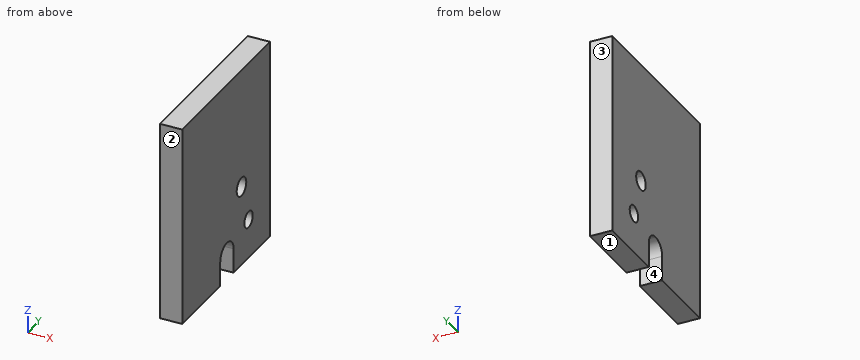
from build123d import *

# Parameters (mm, degrees)
SKETCH_1_W      = 5
SKETCH_1_H      = 5
SKETCH_1_R      = 1.1
EXTRUDE_1_DEPTH = 3
SKETCH_2_W      = 2.809830056
SKETCH_2_H      = 3.158804736
SKETCH_2_H_2    = 9.934341015
EXTRUDE_2_DEPTH = 3


with BuildPart() as part:
    # 草图1 → 凸台-拉伸1 (new body)
    with BuildSketch(Plane(origin=(0, 0, 0), x_dir=(0, 0, -1), z_dir=(1, 0, 0))):
        with Locations((2.5, -2.5)):
            Rectangle(SKETCH_1_W, SKETCH_1_H)
        with Locations((2.5, -2.5)):
            Circle(SKETCH_1_R, mode=Mode.SUBTRACT)
    extrude(amount=EXTRUDE_1_DEPTH)

    # 草图2 → 凸台-拉伸2 (add)
    with BuildSketch(Plane.ZY):
        with Locations((-6.404915028, 1.579402368)):
            Rectangle(SKETCH_2_W, SKETCH_2_H)
        Polygon((-5, 3.158804736), (-5, 0), (0, 0), (19.090169944, 0), (19.090169944, 3.158804736), align=None)
        Polygon((-5, -5), (-5, 0), (-7.809830056, 0), (-7.809830056, -6.406854249), (-5, -6.406854249), align=None)
        with BuildLine():
            Line((0, -5), (-5, -5))
            Line((-5, -5), (-5, -6.406854249))
            Line((-5, -6.406854249), (-4.5, -6.406854249))
            ThreePointArc((-4.5, -6.406854249), (-3.262563133, -6.919417382), (-2.75, -8.156854249))
            ThreePointArc((-2.75, -8.156854249), (-3.262563133, -9.394291117), (-4.5, -9.906854249))
            Line((-4.5, -9.906854249), (-5, -9.906854249))
            Line((-5, -9.906854249), (-5, -19.841195264))
            Line((-5, -19.841195264), (19.090169944, -19.841195264))
            Line((19.090169944, -19.841195264), (19.090169944, -5))
            Line((19.090169944, -5), (4.062297661, -5))
            ThreePointArc((4.062297661, -5), (3, -5.591195264), (1.937702339, -5))
            Line((1.937702339, -5), (0, -5))
        make_face()
        with BuildLine():
            Line((19.090169944, 0), (0, 0))
            Line((0, 0), (0, -5))
            Line((0, -5), (1.937702339, -5))
            ThreePointArc((1.937702339, -5), (2.657488742, -3.139036357), (4.25, -4.341195264))
            ThreePointArc((4.25, -4.341195264), (4.202158907, -4.683706522), (4.062297661, -5))
            Line((4.062297661, -5), (19.090169944, -5))
            Line((19.090169944, -5), (19.090169944, 0))
        make_face()
        with Locations((-6.404915028, -14.874024756)):
            Rectangle(SKETCH_2_W, SKETCH_2_H_2)
    extrude(amount=-EXTRUDE_2_DEPTH)


solid = part.part
The model under review builds one solid part; all positions refer to its coordinate system, in mm. Face numbers are marked on the shaded views. Give positions to 0.01 mm unless a question says otherwise; leave off trailing zeros. Loops run counter-clockwise (first coordinate to the right, second up) from the corner with the lowest first, then second, coordinate; pieces in that order, holes last. Notation, with made-up numbers: (41.5, 15.5) -> (45.5, 15.5) arc R6 ccw to (45.5, 20.5) -> close; hole circle Ø8 at (33.25, -26). An arc over 180 degrees is marked (long way). Put each result on its own line as item: value. Start each with the question number.
1. We need section A-A on z = 3. State the section outline as (x, y) points, then the cut area to 3 significant figures.
2. We need section C-C on y = -2.5. State the section outline as (x, z) points.
3. Wall thickness on probe 1 along Y at (x, z) = (2.95, -3.5); probe 2 along Y at (x, z) = (1.5, -2.5); probe 3 along Y at (x, z) = (0.25, -1.5): over which ranges is each line inside the solid? List them lowest first.
4. We need section D-D on z = -3.25. State the section outline as (x, y) points.
5. Mouldability with a two-part tool opening along Y and no side actions: class the marked faces 1, 2, 3 and 4 as released by +Y, released by -Y, zero draft, split by the parting line, or undercut.
6. We need section B-B on x = 0.45. State the section outline as (y, z) points.
Determined:
1. outline: (0, -19.84) -> (3, -19.84) -> (3, -5.59) -> (0, -5.59) -> close; (0, -3.09) -> (3, -3.09) -> (3, 3.16) -> (0, 3.16) -> close
1. area: 61.5 mm^2
2. outline: (0, -7.81) -> (3, -7.81) -> (3, -3.6) -> (0, -3.6) -> close; (0, -1.4) -> (3, -1.4) -> (3, 19.09) -> (0, 19.09) -> close
3. probe 1: -19.84 to -9.59, -6.72 to -2.96, -2.04 to 3.16
3. probe 2: -19.84 to -3.6, -1.4 to 3.16
3. probe 3: -19.84 to -2.96, -2.04 to 3.16
4. outline: (0, -19.84) -> (3, -19.84) -> (3, -9.38) -> (0, -9.38) -> close; (0, -6.93) -> (3, -6.93) -> (3, -3.3) -> (0, -3.3) -> close; (0, -1.7) -> (3, -1.7) -> (3, 3.16) -> (0, 3.16) -> close
5. face 1: zero draft
5. face 2: released by -Y
5. face 3: released by +Y
5. face 4: undercut
6. outline: (-19.84, -7.81) -> (-9.91, -7.81) -> (-9.91, -4.5) arc R1.75 cw to (-6.41, -4.5) -> (-6.41, -7.81) -> (3.16, -7.81) -> (3.16, 19.09) -> (-19.84, 19.09) -> close; hole circle Ø2.5 at (-4.34, 3); hole circle Ø2.2 at (-2.5, -2.5)
